Autodesk Inventor part; units mm, degrees
ref_plane "YZ Plane" through (0, 0, 0) normal (1, 0, 0) x (0, 1, 0)
ref_plane "XZ Plane" through (0, 0, 0) normal (0, 1, 0) x (-1, 0, 0)
ref_plane "XY Plane" through (0, 0, 0) normal (0, 0, 1) x (1, 0, 0)
sketch "Sketch1" plane through (0, 0, 0) normal (0, 0, 1) x (1, 0, 0)
  line L0 (0, 1489.5) -> (-168.019, 1489.5)
  line L1 (-168.019, 1489.5) -> (-168.019, 0)
  line L2 (-168.019, 0) -> (0, 0)
  line L3 (0, 0) -> (0, 1489.5)
  line L4 (-168.019, 100) -> (-66, 100)
  line L5 (-66, 100) -> (-66, 105)
  line L6 (-66, 105) -> (-168.019, 105)
  line L7 (-168.019, 105) -> (-168.019, 100)
  line L8 (-168.019, 596.6667) -> (-66, 596.6667)
  line L9 (-66, 596.6667) -> (-66, 601.6667)
  line L10 (-66, 601.6667) -> (-168.019, 601.6667)
  line L11 (-168.019, 601.6667) -> (-168.019, 596.6667)
  line L12 (-168.019, 1093.3333) -> (-66, 1093.3333)
  line L13 (-66, 1093.3333) -> (-66, 1098.3333)
  line L14 (-66, 1098.3333) -> (-168.019, 1098.3333)
  line L15 (-168.019, 1098.3333) -> (-168.019, 1093.3333)
  circle A0 centre (-168.019, 1335) radius 30
  point P0 (-168.019, 1098.3333)
  point P1 (-168.019, 1093.3333)
  point P2 (-168.019, 596.6667)
  point P3 (-168.019, 1365)
  point P4 (-168.019, 1305)
  dimension "d0" = 1489.5
  dimension "d1" = 168.019
  dimension "d2" = 5
  dimension "d4" = 100
  dimension "d7" = 496.6667
  dimension "d23" = 66
  dimension "d29" = 60
  dimension "d30" = 1335
extrude "Plate1" add sketch "Sketch1" along normal blind 4 contours L3 L2 L1 L4 L5 L6 L8 L9 L10 L12 L13 L14 A0 L0
chamfer "Corner Chamfer1" distance 3 angle 45 6 edges at (-168.019, 100, 2) (-168.019, 105, 2) (-168.019, 596.6667, 2) (-168.019, 601.6667, 2) (-168.019, 1098.3333, 2) (-168.019, 1093.3333, 2)
equation "\"d0\" = Стрингер_длина"
equation "\"d1\" = стрингер_глубина_3"
equation "\"d2\" = паз_под_стрингер_толщина"
equation "\"d7\" = Шаг_шпангоутов"
equation "\"d23\" = паз_под_стрингер_глубина - Thickness"
equation "\"d29\" = 2 * радиус_выреза_под_сварку"
equation "\"d12\" = Thickness"
equation "\"BendRadius\" = Thickness"
equation "\"BendReliefWidth\" = Thickness"
equation "\"BendReliefDepth\" = 0.5 * Thickness"
equation "\"CornerReliefSize\" = 4 * Thickness"
equation "\"MinimumRemnant\" = 2 * Thickness"
equation "\"TransitionRadius\" = BendRadius"
equation "\"JacobiRadiusSize\" = BendRadius"
equation "\"GapSize\" = Thickness"
properties part number "GBK 3115 stringer 3" material "Steel"
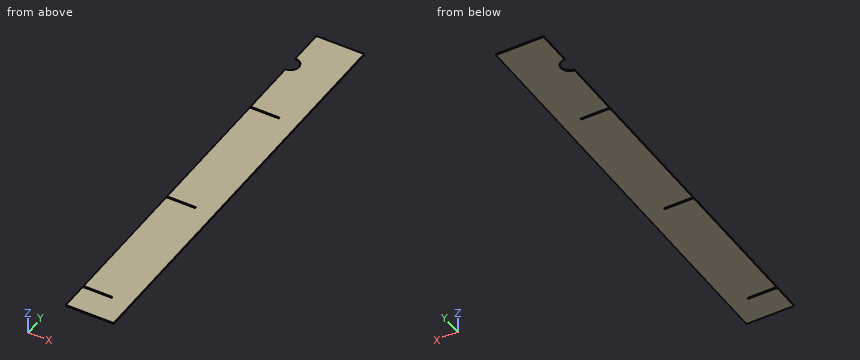
Check sheet for the modelled part. Datum: model origin and axes. Units: mm. Give positions to 0.01 mm unless a question says otherwise; leave off trailing zeros. Loops run counter-clockwise (first coordinate to the right, second up) from the corner with the lowest first, then second, coordinate; pieces in that order, holes last. Notation, with made-up numbers: (6, 2.5) - (45, 2.5) arc R23 ccw to (45, 39.5) - close; hole circle Ø3 at (24.5, 4.25). An arc over 180 degrees is marked (long way). One line per question, with ' | ' between items. Start each with the question number.
1. Material ranges on line 1 along Y through (x, z) = (-85.5, 0.35); line 2 along Y through (x, z) = (-156, 0.7); line 3 along Y through (x, z) = (-160.5, 0.35), recorded low to high. Write a range as [from, to].
2. Cross-section at A-A, the plane y = 1335. Enter the section's corners in (x, z), plus the area to 3 significant figures.
3. Gauge pin test, flat end, axial feed: pin 1 Ø1.2 at (y, z) = (102, 2.5) entering from -X. Record the tip position at first contact, or that the pin passes through.
Check result:
1) line 1: y = [0, 100], [105, 596.67], [601.67, 1093.33], [1098.33, 1489.5] | line 2: y = [0, 100], [105, 596.67], [601.67, 1093.33], [1098.33, 1307.51], [1362.49, 1489.5] | line 3: y = [0, 100], [105, 596.67], [601.67, 1093.33], [1098.33, 1305.96], [1364.04, 1489.5]
2) outline: (-138.02, 0) - (0, 0) - (0, 4) - (-138.02, 4) - close | area: 552 mm2
3) pin 1: stops at x = -66
